Drawing for the job (mm, zero at the part's lowest x, y, z). Coordinates: 2 decimals unless noted, no trailing zeros. Loops run counter-clockwise (first coordinate to the right, second up) from the corner with the lowest first, then second, coordinate; pieces in that order, holes last. Notation, with made-up numbers: (3, 73) -> (49, 73) arc R19 ccw to (49, 99) -> close; hole circle Ø5 at (51, 48.25). An arc over 180 degrees is marked (long way). Write each question's results on one line, items separated by ' | '.
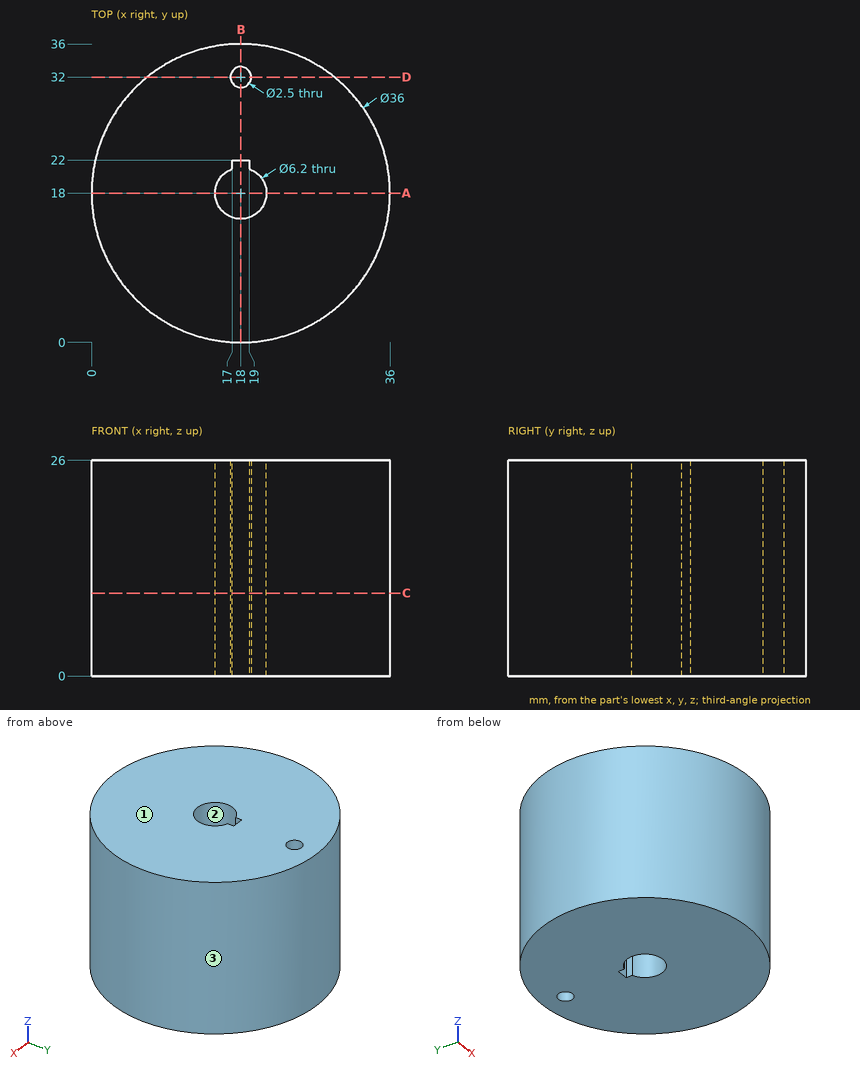
1) Slice it at D-D (y = 32). Write the cut outline in (x, z).
Outcome:
outline: (6.69, 0) -> (16.75, 0) -> (16.75, 26) -> (6.69, 26) -> close; (19.25, 0) -> (29.31, 0) -> (29.31, 26) -> (19.25, 26) -> close
2) Slice it at C-C (z = 10). Write the cut outline in (x, y), then the cut area to 3 significant figures.
Outcome:
outline: circle Ø36 at (18, 18); hole circle Ø2.5 at (18, 32); hole (17, 20.93) arc R3.1 ccw (long way) to (19, 20.93) -> (19, 22) -> (17, 22) -> close | area: 981 mm^2
3) Pin check, flat tips, straight feed: pin 1 (1 mm diameter, centred on x = 14.5, z = 22.5, fed in from +Y); pin 2 (1.5 mm diameter, centred on y = 31, z = 17, fed in from +X); pin 3 (1.2 mm diameter, centred on y = 21.5, z = 15.5, fed in from -X); pin 4 (5.5 mm diameter, centred on x = 18, y = 18, fed in from +Z). Stop position of each tip, or through.
Outcome:
pin 1: stops at y = 35.75 | pin 2: stops at x = 31.19 | pin 3: stops at x = 0.24 | pin 4: passes through
4) Slice it at A-A (y = 18). Write the cut outline in (x, z).
Outcome:
outline: (0, 0) -> (14.9, 0) -> (14.9, 26) -> (0, 26) -> close; (21.1, 0) -> (36, 0) -> (36, 26) -> (21.1, 26) -> close
5) Drill centre lines: L1, parallel to Y at x = 18, z = 15.25; L2, parallel to Y at x = 16.5, z = 12; L3, parallel to X at y = 32, z = 8.5. Where is each one in solid material? Low to high. Write a range as from..to.
Outcome:
L1: y = 0..14.9, 22..30.75, 33.25..36 | L2: y = 0.06..15.29, 20.71..35.94 | L3: x = 6.69..16.75, 19.25..29.31
6) Two-plate mould, pull along X, no slides. Class the marked faces 1, 2 and 3: pulls with the +X half, pulls with the -X half, needs draft (parallel to the pull), parting line crosses it, or undercut.
Outcome:
face 1: needs draft | face 2: undercut | face 3: parting line crosses it
7) Slice it at B-B (x = 18). Write the cut outline in (y, z).
Outcome:
outline: (0, 0) -> (14.9, 0) -> (14.9, 26) -> (0, 26) -> close; (22, 0) -> (30.75, 0) -> (30.75, 26) -> (22, 26) -> close; (33.25, 0) -> (36, 0) -> (36, 26) -> (33.25, 26) -> close
